Check sheet for the modelled part. Datum: model origin and axes. Units: mm. Give positions to 0.01 mm unless a question says otherwise; leave off trailing zeros. Order: outer loops, then holes, each group sorted by start corner. A loop starts at its lowest first (then second) coordinate and runs counter-clockwise, first axis right, second up.
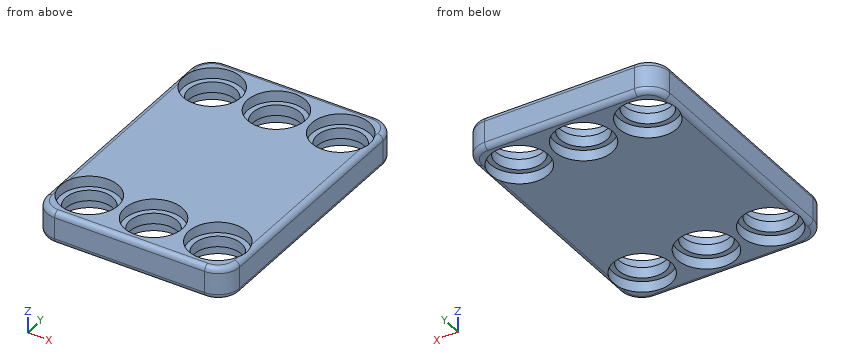
from build123d import *

# Parameters (mm, degrees)
SKETCH1_W           = 18
SKETCH1_H           = 25
BOSS_EXTRUDE1_DEPTH = 3
HOLE1_D             = 4.4
HOLE1_DEPTH         = 100
HOLE1_CBORE_D       = 5.4
HOLE1_CBORE_DEPTH   = 1
HOLE2_D             = 4.4
HOLE2_DEPTH         = 100
HOLE2_CBORE_D       = 5.4
HOLE2_CBORE_DEPTH   = 1
FILLET1_R           = 2
FILLET2_R           = 0.5


with BuildPart() as part:
    # Sketch1 → Boss-Extrude1 (new body)
    with BuildSketch(Plane.XY):
        with Locations((0, -9)):
            Rectangle(SKETCH1_W, SKETCH1_H)
    extrude(amount=BOSS_EXTRUDE1_DEPTH)

    # Hole1
    with Locations(Plane.XY.offset(3)):
        with Locations((-6, 0), (0, 0), (6, 0), (-6, -18), (0, -18), (6, -18)):
            CounterBoreHole(HOLE1_D / 2, HOLE1_CBORE_D / 2, HOLE1_CBORE_DEPTH, depth=HOLE1_DEPTH)

    # Hole2
    with Locations(Plane(origin=(0, 0, 0), x_dir=(-1, 0, 0), z_dir=(0, 0, -1))):
        with Locations((-6, 0), (0, 0), (6, 0), (6, -18), (0, -18), (-6, -18)):
            CounterBoreHole(HOLE2_D / 2, HOLE2_CBORE_D / 2, HOLE2_CBORE_DEPTH, depth=HOLE2_DEPTH)

    # Fillet1
    fillet1_edges = [part.edges().sort_by_distance(p)[0] for p in [
        (9, -21.5, 1.5),
        (-9, -21.5, 1.5),
        (-9, 3.5, 1.5),
        (9, 3.5, 1.5),
    ]]
    fillet(fillet1_edges, radius=FILLET1_R)

    # Fillet2
    # the kernel refuses this fillet: 0.5 mm, written as the material it takes off along each edge
    with BuildSketch(Plane(origin=(9, -19.5, 0), x_dir=(-1, 0, 0), z_dir=(0, 1, 0)), Plane(origin=(-9, 1.5, 0), x_dir=(1, 0, 0), z_dir=(0, -1, 0))) as fillet2_piece_1:
        with BuildLine():
            CenterArc((FILLET2_R, FILLET2_R), FILLET2_R, 180, 90)
            Line((0, FILLET2_R), (0, 0))
            Line((0, 0), (FILLET2_R, 0))
        make_face()
    extrude(amount=21, mode=Mode.SUBTRACT)
    with BuildSketch(Plane(origin=(9, -19.5, 3), x_dir=(-1, 0, 0), z_dir=(0, 1, 0)), Plane(origin=(-9, 1.5, 3), x_dir=(1, 0, 0), z_dir=(0, -1, 0))) as fillet2_piece_2:
        with BuildLine():
            CenterArc((FILLET2_R, -FILLET2_R), FILLET2_R, 90, 90)
            Line((0, -FILLET2_R), (0, 0))
            Line((0, 0), (FILLET2_R, 0))
        make_face()
    extrude(amount=21, mode=Mode.SUBTRACT)
    with BuildSketch(Plane(origin=(-7, -21.5, 0), x_dir=(0, 1, 0), z_dir=(1, 0, 0)), Plane(origin=(7, 3.5, 3), x_dir=(0, 0, -1), z_dir=(-1, 0, 0))) as fillet2_piece_3:
        with BuildLine():
            CenterArc((FILLET2_R, FILLET2_R), FILLET2_R, 180, 90)
            Line((0, FILLET2_R), (0, 0))
            Line((0, 0), (FILLET2_R, 0))
        make_face()
    extrude(amount=14, mode=Mode.SUBTRACT)
    with BuildSketch(Plane(origin=(7, 3.5, 0), x_dir=(0, 0, 1), z_dir=(-1, 0, 0)), Plane(origin=(-7, -21.5, 3), x_dir=(0, 1, 0), z_dir=(1, 0, 0))) as fillet2_piece_4:
        with BuildLine():
            CenterArc((FILLET2_R, -FILLET2_R), FILLET2_R, 90, 90)
            Line((0, -FILLET2_R), (0, 0))
            Line((0, 0), (FILLET2_R, 0))
        make_face()
    extrude(amount=14, mode=Mode.SUBTRACT)
    with BuildSketch(Plane(origin=(7, 1.5, 0), x_dir=(0, 1, 0), z_dir=(-1, 0, 0))) as fillet2_piece_5:
        with BuildLine():
            CenterArc((2 - FILLET2_R, -FILLET2_R), FILLET2_R, 0, 90)
            Line((2, -FILLET2_R), (2, 0))
            Line((2, 0), (2 - FILLET2_R, 0))
        make_face()
    revolve(axis=Axis((7, 1.5, 0), (0, 0, -1)), revolution_arc=90, mode=Mode.SUBTRACT)
    with BuildSketch(Plane(origin=(-7, 1.5, 0), x_dir=(0, 1, 0), z_dir=(1, 0, 0))) as fillet2_piece_6:
        with BuildLine():
            CenterArc((2 - FILLET2_R, FILLET2_R), FILLET2_R, 270, 90)
            Line((2, FILLET2_R), (2, 0))
            Line((2, 0), (2 - FILLET2_R, 0))
        make_face()
    revolve(axis=Axis((-7, 1.5, 0), (0, 0, 1)), revolution_arc=90, mode=Mode.SUBTRACT)
    with BuildSketch(Plane(origin=(-7, -19.5, 0), x_dir=(0, -1, 0), z_dir=(1, 0, 0))) as fillet2_piece_7:
        with BuildLine():
            CenterArc((2 - FILLET2_R, -FILLET2_R), FILLET2_R, 0, 90)
            Line((2, -FILLET2_R), (2, 0))
            Line((2, 0), (2 - FILLET2_R, 0))
        make_face()
    revolve(axis=Axis((-7, -19.5, 0), (0, 0, -1)), revolution_arc=90, mode=Mode.SUBTRACT)
    with BuildSketch(Plane(origin=(7, -19.5, 0), x_dir=(0, -1, 0), z_dir=(-1, 0, 0))) as fillet2_piece_8:
        with BuildLine():
            CenterArc((2 - FILLET2_R, FILLET2_R), FILLET2_R, 270, 90)
            Line((2, FILLET2_R), (2, 0))
            Line((2, 0), (2 - FILLET2_R, 0))
        make_face()
    revolve(axis=Axis((7, -19.5, 0), (0, 0, 1)), revolution_arc=90, mode=Mode.SUBTRACT)
    with BuildSketch(Plane(origin=(7, 1.5, 3), x_dir=(0, 1, 0), z_dir=(-1, 0, 0))) as fillet2_piece_9:
        with BuildLine():
            CenterArc((2 - FILLET2_R, FILLET2_R), FILLET2_R, 270, 90)
            Line((2 - FILLET2_R, 0), (2, 0))
            Line((2, 0), (2, FILLET2_R))
        make_face()
    revolve(axis=Axis((7, 1.5, 3), (0, 0, -1)), revolution_arc=90, mode=Mode.SUBTRACT)
    with BuildSketch(Plane(origin=(-7, 1.5, 3), x_dir=(0, 1, 0), z_dir=(1, 0, 0))) as fillet2_piece_10:
        with BuildLine():
            CenterArc((2 - FILLET2_R, -FILLET2_R), FILLET2_R, 0, 90)
            Line((2 - FILLET2_R, 0), (2, 0))
            Line((2, 0), (2, -FILLET2_R))
        make_face()
    revolve(axis=Axis((-7, 1.5, 3), (0, 0, 1)), revolution_arc=90, mode=Mode.SUBTRACT)
    with BuildSketch(Plane(origin=(-7, -19.5, 3), x_dir=(0, -1, 0), z_dir=(1, 0, 0))) as fillet2_piece_11:
        with BuildLine():
            CenterArc((2 - FILLET2_R, FILLET2_R), FILLET2_R, 270, 90)
            Line((2, FILLET2_R), (2, 0))
            Line((2, 0), (2 - FILLET2_R, 0))
        make_face()
    revolve(axis=Axis((-7, -19.5, 3), (0, 0, -1)), revolution_arc=90, mode=Mode.SUBTRACT)
    with BuildSketch(Plane(origin=(7, -19.5, 3), x_dir=(0, -1, 0), z_dir=(-1, 0, 0))) as fillet2_piece_12:
        with BuildLine():
            CenterArc((2 - FILLET2_R, -FILLET2_R), FILLET2_R, 0, 90)
            Line((2, -FILLET2_R), (2, 0))
            Line((2, 0), (2 - FILLET2_R, 0))
        make_face()
    revolve(axis=Axis((7, -19.5, 3), (0, 0, 1)), revolution_arc=90, mode=Mode.SUBTRACT)


solid = part.part
1) Section check A-A, the plane z = 2.25. Record the cut outline in (x, y).
Recorded:
outline: (-9, -19.5) arc R2 ccw to (-7, -21.5) - (7, -21.5) arc R2 ccw to (9, -19.5) - (9, 1.5) arc R2 ccw to (7, 3.5) - (-7, 3.5) arc R2 ccw to (-9, 1.5) - close; hole circle Ø5.4 at (-6, -18); hole circle Ø5.4 at (-6, 0); hole circle Ø5.4 at (0, -18); hole circle Ø5.4 at (0, 0); hole circle Ø5.4 at (6, -18); hole circle Ø5.4 at (6, 0)
2) Material ranges on L1, parallel to Y at x = -6, z = 0.5; L2, parallel to X at y = -16.75, z = 0.2; L3, parallel to Y at x = 1.5, z = 2.7 (3 decimals), recorded low to high.
Recorded:
L1: y = -21.5 to -20.7, -15.3 to -2.7, 2.7 to 3.5
L2: x = -8.9 to -8.39, -3.61 to -2.39, 2.39 to 3.61, 8.39 to 8.9
L3: y = -21.458 to -20.245, -15.755 to -2.245, 2.245 to 3.458
3) Depth check by flat-ended pin: pin 1 Ø7 at (x, y) = (-6, 0) entering from +Z; pin 2 Ø4.5 at (x, y) = (6, 0) entering from -Z; pin 3 Ø5 at (x, y) = (-6, -18) entering from +Z. Enter the tip coordinate at first touch or a pass-through.
Recorded:
pin 1: stops at z = 3
pin 2: stops at z = 1
pin 3: stops at z = 2
4) Section check B-B, the plane x = 0. State how many separate pieces and enclosed holes the cut face has, then the cut area to 3 significant figures.
Recorded:
separate pieces: 3
enclosed holes: 0
area: 44.4 mm2
